Geometry: final body of the model. Coordinates: model frame, mm. A direction names the side the tool comes from. Coordinates: 2 decimals unless noted, no trailing zeros. Order: outer loops, then holes, each group sorted by start corner. A loop starts at its lowest first (then second) coordinate and runs counter-clockwise, first axis right, second up. Notation, with made-up numbers: M 70,-27 L 124,-27 A10 ccw 124,-18 Z; hole C 20.25,3 d11. An arc over 180 degrees is marked long. Use CSV: the item, a comma, the result in double quotes. Start each with the question number.
1. Section query A-A on y = -24. Return the cut outline in (x, z).
2. Set-up query: faces 1 (the flat face through (-1, 60, 5)), 2 (the flat face through (-8.949, -9, 5)). Return all of +Z, -Z, +X, -X, +Y, -Y with unobstructed straight access to the full face (end or side cutting, diameter ignored); none if empty.
3. Material intervals for line 1 (X direction, y = 19.5, z = 7); line 2 (Y direction, x = 8, z = 1.25); line 3 (Y direction, x = -24, z = 7.75), sorted ascending.
4. Pull-direction query (Y, two-part tool) for faces 3 (the flat face through (-24.18, 41.55, 5.07)), 4 (the cylindrical face through (-56.99, -57.15, 4.93)), 5 (the flat face through (14, 1, 0)), 6 (the cylindrical face through (56.99, 57.15, 4.93)); classes: pulls with the +Y half, pulls with the -Y half, needs draft (parallel to the pull), parting line crosses it, or undercut.
5. Section query B-B on z = 3.5. Return the cut outline in (x, y), and give its area (3 significant figures).
6. Section query C-C on x = -26. Return the cut outline in (y, z).
from build123d import *

# Parameters (mm, degrees)
BOSS_EXTRUDE1_DEPTH = 10
CUT_EXTRUDE2_DEPTH  = 10


with BuildPart() as part:
    # Sketch1 → Boss-Extrude1 (new body)
    with BuildSketch(Plane.XY):
        with BuildLine():
            Line((-50, 60), (50, 60))
            ThreePointArc((50, 60), (57.071067812, 57.071067812), (60, 50))
            Line((60, 50), (60, -50))
            ThreePointArc((60, -50), (57.071067812, -57.071067812), (50, -60))
            Line((50, -60), (-50, -60))
            ThreePointArc((-50, -60), (-57.071067812, -57.071067812), (-60, -50))
            Line((-60, -50), (-60, 50))
            ThreePointArc((-60, 50), (-57.071067812, 57.071067812), (-50, 60))
        make_face()
    extrude(amount=BOSS_EXTRUDE1_DEPTH)

    # Sketch2 → Cut-Extrude2 (cut)
    with BuildSketch(Plane.XY.offset(10)):
        Polygon((-18.744391026, 50), (9, 50), (9, -50), (-8.948717949, -50), (-8.948717949, 33.333333333), (-29.461538462, 33.333333333), align=None)
    extrude(amount=-CUT_EXTRUDE2_DEPTH, mode=Mode.SUBTRACT)


solid = part.part
Results list:
1,outline,"M -60,0 L -8.95,0 L -8.95,10 L -60,10 Z; M 9,0 L 60,0 L 60,10 L 9,10 Z"
2,face 1,"+Z, -Z, +X, -X, +Y"
2,face 2,"+Z, -Z"
3,line 1,"x = -60 to -8.95, 9 to 60"
3,line 2,"y = -60 to -50, 50 to 60"
3,line 3,"y = -60 to 33.33, 41.83 to 60"
4,face 3,"undercut"
4,face 4,"pulls with the -Y half"
4,face 5,"needs draft"
4,face 6,"pulls with the +Y half"
5,outline,"M -60,-50 A10 ccw -50,-60 L 50,-60 A10 ccw 60,-50 L 60,50 A10 ccw 50,60 L -50,60 A10 ccw -60,50 Z; hole M -29.46,33.33 L -8.95,33.33 L -8.95,-50 L 9,-50 L 9,50 L -18.74,50 Z"
5,area,"12,300 mm²"
6,outline,"M -60,0 L 33.33,0 L 33.33,10 L -60,10 Z; M 38.72,0 L 60,0 L 60,10 L 38.72,10 Z"
